Can you work these out from the model? Positions are in its coordinate system, mm. A direction names the side the tool comes from. Give positions to 0.01 mm unless a question says otherwise; leave off trailing zeros. Loops run counter-clockwise (first coordinate to the right, second up) from the corner with the lowest first, then second, coordinate; pieces in that order, holes last. Notation, with made-up numbers: (75.5, 8) -> (108.5, 8) arc R31 ccw to (108.5, 42) -> close; hole circle Ø6 at (1, -21.75). An arc over 180 degrees is marked (long way). One line per question, with ' | ' between items.
from build123d import *

# Parameters (mm, degrees)
SKETCH_1_R          = 18.5
EXTRUDE_1_DEPTH     = 44
SKETCH_2_R          = 2.75
EXTRUDE_2_DEPTH     = 22
SKETCH_3_R          = 1
CUT_EXTRUDE_1_DEPTH = 1


with BuildPart() as part:
    # 草图1 → 凸台-拉伸1 (new body)
    with BuildSketch(Plane.XY):
        Circle(SKETCH_1_R)
    extrude(amount=EXTRUDE_1_DEPTH)

    # 草图2 → 凸台-拉伸2 (add)
    with BuildSketch(Plane.XY.offset(44)):
        with Locations((0, 6.5)):
            Circle(SKETCH_2_R)
    extrude(amount=EXTRUDE_2_DEPTH)

    # 草图3 → 切除-拉伸1 (cut)
    with BuildSketch(Plane.XY.offset(44)):
        with Locations((0, -10)):
            Circle(SKETCH_3_R)
    extrude(amount=-CUT_EXTRUDE_1_DEPTH, mode=Mode.SUBTRACT)


solid = part.part
Q1. If we section it at A-A (x = 0): Write out the boundary of the cut face in (y, z).
Entries:
outline: (-18.5, 0) -> (18.5, 0) -> (18.5, 44) -> (9.25, 44) -> (9.25, 66) -> (3.75, 66) -> (3.75, 44) -> (-9, 44) -> (-9, 43) -> (-11, 43) -> (-11, 44) -> (-18.5, 44) -> close
Q2. If we mould it in two halves opening along X, with no side actions, what happens to faces 3 (the face through (0, 0, 0)), 4 (the face through (-0.13, -9.01, 43.51)), 5 (the face through (0, -10, 43)), 6 (the face through (-4.01, -18.06, 21.69))? For each: pulls with the +X half, pulls with the -X half, needs draft (parallel to the pull), parting line crosses it, or undercut.
Entries:
face 3: needs draft | face 4: undercut | face 5: undercut | face 6: parting line crosses it
Q3. On a 3-axis mill with a long thin cutter (end or side, diameter ignored), from which of +Z, -Z, +X, -X, +Y, -Y can I reach the whole of each face in a straight line? I mean faces 1 (the face through (0, 7, 66)), 2 (the face through (-0.596, 3.815, 54.846)). Say none if no direction works.
Entries:
face 1: +Z, +X, -X, +Y, -Y | face 2: +Z
Q4. If we section it at C-C (z = 38.5): Write out the boundary of the cut face in (x, y), plus the area to 3 significant figures.
Entries:
outline: circle Ø37 at (0, 0) | area: 1,080 mm²
Q5. If we section it at B-B (y = -10): Write out the boundary of the cut face in (x, z), plus the area to 3 significant figures.
Entries:
outline: (-15.56, 0) -> (15.56, 0) -> (15.56, 44) -> (1, 44) -> (1, 43) -> (-1, 43) -> (-1, 44) -> (-15.56, 44) -> close | area: 1,370 mm²
Q6. For pin 1 Ø10 at (x, z) = (6, 41.5) entering from +Y; pin 2 Ø11 at (x, y) = (7.5, 6) entering from +Z; pin 3 Ø2 at (x, y) = (0.5, -10) entering from +Z; pin 4 Ø1.6 at (x, y) = (0, -10) entering from +Z, each with a flat end and sliding along its axis, tell me the tip position at first contact or that it passes through.
Entries:
pin 1: y = 18.47 | pin 2: z = 66 | pin 3: z = 44 | pin 4: z = 43
Q7. If I drill on probe 1 along Y at (x, z) = (0, 43.3); probe 2 along Z at (x, y) = (-6, 9); probe 3 along Y at (x, z) = (-15.5, 18.5), over which ranges is the centre line in solid material (lowest first)? Write a range as from..to.
Entries:
probe 1: -18.5..-11, -9..18.5 | probe 2: 0..44 | probe 3: -10.1..10.1
Q8. If we section it at D-D (y = 6.5): Write out the boundary of the cut face in (x, z).
Entries:
outline: (-17.32, 0) -> (17.32, 0) -> (17.32, 44) -> (2.75, 44) -> (2.75, 66) -> (-2.75, 66) -> (-2.75, 44) -> (-17.32, 44) -> close
